For this review, take the finished solid that the model builds, in its own axes (mm). Face numbers are marked on the shaded views. A direction names the side the tool comes from. Coordinates: 2 decimals unless noted, no trailing zeros. Write each loop counter-clockwise with the first axis right and the second up, starting at its lowest first coordinate (ties: lowest second). Pieces come first, ordered by that corner, then holes.
1) Insertion check: P1, Ø1.5, axis at y = 10, z = 10, coming from the +X side; P2, Ø2.5, axis at x = 10.5, y = 1, coming from the +Z side; P3, Ø2.5, axis at y = 10, z = 10.5, coming from the -X side. Each pin has a flat end and moves straight along its axis. Give the tip position at first contact, or say it passes through.
2) We need section D-D on x = -10. Write out the cut boundary in (y, z).
3) Mouldability with a two-part tool opening along Y and no side actions: class the marked faces 1, 2 and 3 as pulls with the +Y half, pulls with the -Y half, needs draft (parallel to the pull), parting line crosses it, or undercut.
4) We need section A-A on x = 0. Write out the cut boundary in (y, z), then the cut area to 3 significant figures.
5) We need section C-C on z = 4. Write out the cut boundary in (x, y), then the cut area to 3 significant figures.
6) For the marked faces 4, 5 and 6, list the 3-axis set-ups (+Z, -Z, +X, -X, +Y, -Y) from which the entire face can be reached by the end or side of a thin tool; tool diameter is ignored.
7) To check wall thickness, follow line 1 along Y through (x, z) = (0, 2.55); line 2 along Y through (x, z) = (0, 7.5); line 3 along X through (y, z) = (-2.5, 6.25). State the ranges of each line that lie inside material, in increasing order.
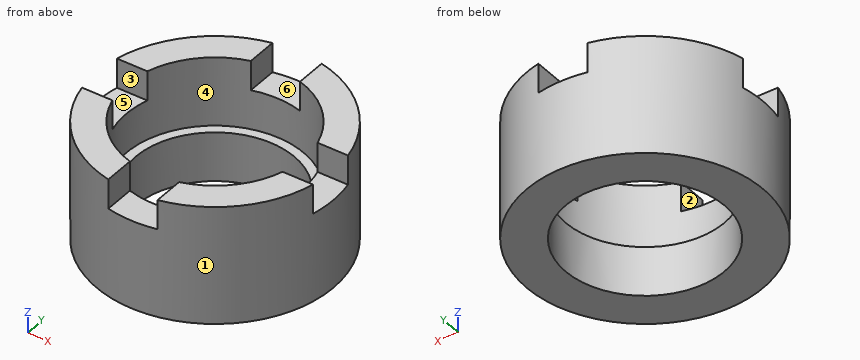
from build123d import *

# Parameters (mm, degrees)
SKETCH_1_R          = 12
SKETCH_1_R_2        = 8.05
EXTRUDE_1_DEPTH     = 12
CUT_EXTRUDE_1_DEPTH = 3
SKETCH_4_R          = 9
CUT_EXTRUDE_2_DEPTH = 7


with BuildPart() as part:
    # 草图1 → 凸台-拉伸1 (new body)
    with BuildSketch(Plane.XY):
        Circle(SKETCH_1_R)
        Circle(SKETCH_1_R_2, mode=Mode.SUBTRACT)
    extrude(amount=EXTRUDE_1_DEPTH)

    # 草图3 → 切除-拉伸1 (cut)
    with BuildSketch(Plane.XY.offset(12)):
        Polygon((-16.5, 2.5), (-2.5, 2.5), (-2.5, 16.5), (2.5, 16.5), (2.5, 2.5), (16.5, 2.5), (16.5, -2.5), (2.5, -2.5), (2.5, -16.5), (-2.5, -16.5), (-2.5, -2.5), (-16.5, -2.5), align=None)
    extrude(amount=-CUT_EXTRUDE_1_DEPTH, mode=Mode.SUBTRACT)

    # 草图4 → 切除-拉伸2 (cut)
    with BuildSketch(Plane.XY.offset(12)):
        Circle(SKETCH_4_R)
    extrude(amount=-CUT_EXTRUDE_2_DEPTH, mode=Mode.SUBTRACT)


solid = part.part
Result:
1. P1: stops at x = 7.64
1. P2: stops at z = 9
1. P3: stops at x = -8.21
2. outline: (-6.63, 0) - (6.63, 0) - (6.63, 12) - (2.5, 12) - (2.5, 9) - (-2.5, 9) - (-2.5, 12) - (-6.63, 12) - close
3. face 1: parting line crosses it
3. face 2: needs draft
3. face 3: undercut
4. outline: (-12, 0) - (-8.05, 0) - (-8.05, 5) - (-9, 5) - (-9, 9) - (-12, 9) - close; (8.05, 0) - (12, 0) - (12, 9) - (9, 9) - (9, 5) - (8.05, 5) - close
4. area: 63.5 mm2
5. outline: circle Ø24 at (0, 0); hole circle Ø16.1 at (0, 0)
5. area: 249 mm2
6. face 4: +Z
6. face 5: +Z, +X, -X
6. face 6: +Z, +Y, -Y
7. line 1: y = -12 to -8.05, 8.05 to 12
7. line 2: y = -12 to -9, 9 to 12
7. line 3: x = -11.74 to -8.65, 8.65 to 11.74
